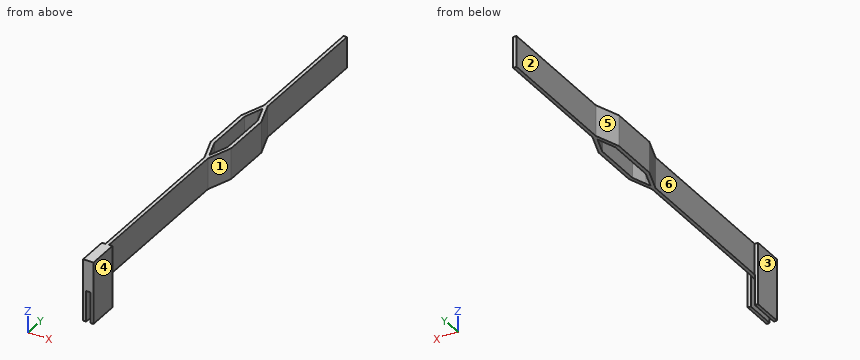
from build123d import *

# Parameters (mm, degrees)
F1_DEPTH = 4.5
F2_W     = 0.5
F2_H     = 4.5
F3_DEPTH = 9
F4_W     = 0.05
F4_H     = 4.5
F5_DEPTH = 25


with BuildPart() as f1:
    # F0 (on Top) → F1 (new body)
    with BuildSketch(Plane.XY):
        Polygon((-0.469149, 27.706926), (-0.969149, 27.706926), (-0.969149, 8.820471), (-2.198889, 5.306926), (-2.198889, -1.893074), (-0.969149, -5.406618), (-0.969149, -33.493074), (-0.469149, -33.493074), (-0.469149, -5.406618), (0.760592, -1.893074), (0.760592, 5.306926), (-0.469149, 8.820471), align=None)
        Polygon((-1.669149, -1.893074), (-1.669149, 5.306926), (-0.969149, 7.306926), (-0.719149, 8.021212), (-0.469149, 7.306926), (0.230851, 5.306926), (0.230851, -1.893074), (-0.469149, -3.893074), (-0.719149, -4.607359), (-0.969149, -3.893074), align=None, mode=Mode.SUBTRACT)
    extrude(amount=F1_DEPTH)

    # F2 (on face) → F3 (join)
    with BuildSketch(Plane.XY.offset(4.5)):
        with Locations((-1.219149, -31.243074)):
            Rectangle(F2_W, F2_H)
        with Locations((-0.219149, -31.243074)):
            Rectangle(F2_W, F2_H)
    extrude(amount=-F3_DEPTH)

    # F4 (on face) → F5 (cut)
    with BuildSketch(Plane(origin=(0, 0, 0), x_dir=(1, 0, 0), z_dir=(0, 0, -1))):
        with Locations((-0.994149, 31.243074)):
            Rectangle(F4_W, F4_H)
        with Locations((-0.444149, 31.243074)):
            Rectangle(F4_W, F4_H)
    extrude(amount=F5_DEPTH, mode=Mode.SUBTRACT)


solid = f1.part
Work out the finished part from the listing and answer in its coordinate system (mm). Face numbers are marked on the shaded views. A direction names the side the tool comes from. Give positions to 0.01 mm unless a question says otherwise; leave off trailing zeros. Order: outer loops, then holes, each group sorted by start corner. A loop starts at its lowest first (then second) coordinate and runs counter-clockwise, first axis right, second up. Notation, with made-up numbers: (26.5, 44.25) -> (49.5, 44.25) arc R18 cw to (49.5, 59.25) -> close; hole circle Ø1 at (-25.5, 44). An arc over 180 degrees is marked (long way). One line per item, written item: value.
Item 1: Straight lines are drawn through the part: probe 1 along Y at (x, z) = (-1.05, -0.5); probe 2 along X at (y, z) = (-9.5, 1.5); probe 3 along Z at (x, y) = (0.5, 3). For each, find the intervals that lie inside material, in ascending order.
Answer sheet:
probe 1: -33.49 to -28.99
probe 2: -0.97 to -0.47
probe 3: 0 to 4.5
Item 2: A tool of negligible diameter and unlimited length cuts with its end or side. For the marked faces 1, 2 and 3, from which of +Z, -Z, +X, -X, +Y, -Y can it reach the whole face along a straight path? Write none if from no direction.
Answer sheet:
face 1: +Z, -Z, +X
face 2: +Z, -Z, -X, +Y
face 3: +Z, -Z, -X, -Y
Item 3: Determine the mould class of the marked faces 4, 5 and 6 for opening direction Y: released by +Y, released by -Y, zero draft, split by the parting line, or undercut.
Answer sheet:
face 4: zero draft
face 5: released by +Y
face 6: undercut
Item 4: Find section B-B, the plane z = 1.25. Give the vertices of the cut face in (x, y).
Answer sheet:
outline: (-2.2, -1.89) -> (-0.97, -5.41) -> (-0.97, -28.99) -> (-1.47, -28.99) -> (-1.47, -33.49) -> (0.03, -33.49) -> (0.03, -28.99) -> (-0.47, -28.99) -> (-0.47, -5.41) -> (0.76, -1.89) -> (0.76, 5.31) -> (-0.47, 8.82) -> (-0.47, 27.71) -> (-0.97, 27.71) -> (-0.97, 8.82) -> (-2.2, 5.31) -> close; hole (-1.67, -1.89) -> (-0.97, -3.89) -> (-0.72, -4.61) -> (-0.47, -3.89) -> (0.23, -1.89) -> (0.23, 5.31) -> (-0.47, 7.31) -> (-0.72, 8.02) -> (-0.97, 7.31) -> (-1.67, 5.31) -> close
Item 5: Find section A-A, the plane z = -2. Give the vertices of the cut face in (x, y), plus the area to 3 significant figures.
Answer sheet:
outline: (-1.47, -33.49) -> (-1.02, -33.49) -> (-1.02, -28.99) -> (-1.47, -28.99) -> close; (-0.42, -33.49) -> (0.03, -33.49) -> (0.03, -28.99) -> (-0.42, -28.99) -> close
area: 4.05 mm²
Item 6: Flat-ended cylindrical pins translate along their axes: P1, Ø2, axis at y = 20, z = 1.5, coming from the -X side; P2, Ø2, axis at y = 17.5, z = 1.5, coming from the +X side; P3, Ø2, axis at y = -32.5, z = -1.5, coming from the -X side. Find the tip coordinate at first contact, or state that the pin passes through.
Answer sheet:
P1: x = -0.97
P2: x = -0.47
P3: x = -1.47
Item 7: Find section C-C, the plane y = 10. Give the vertices of the cut face in (x, z).
Answer sheet:
outline: (-0.97, 0) -> (-0.47, 0) -> (-0.47, 4.5) -> (-0.97, 4.5) -> close
